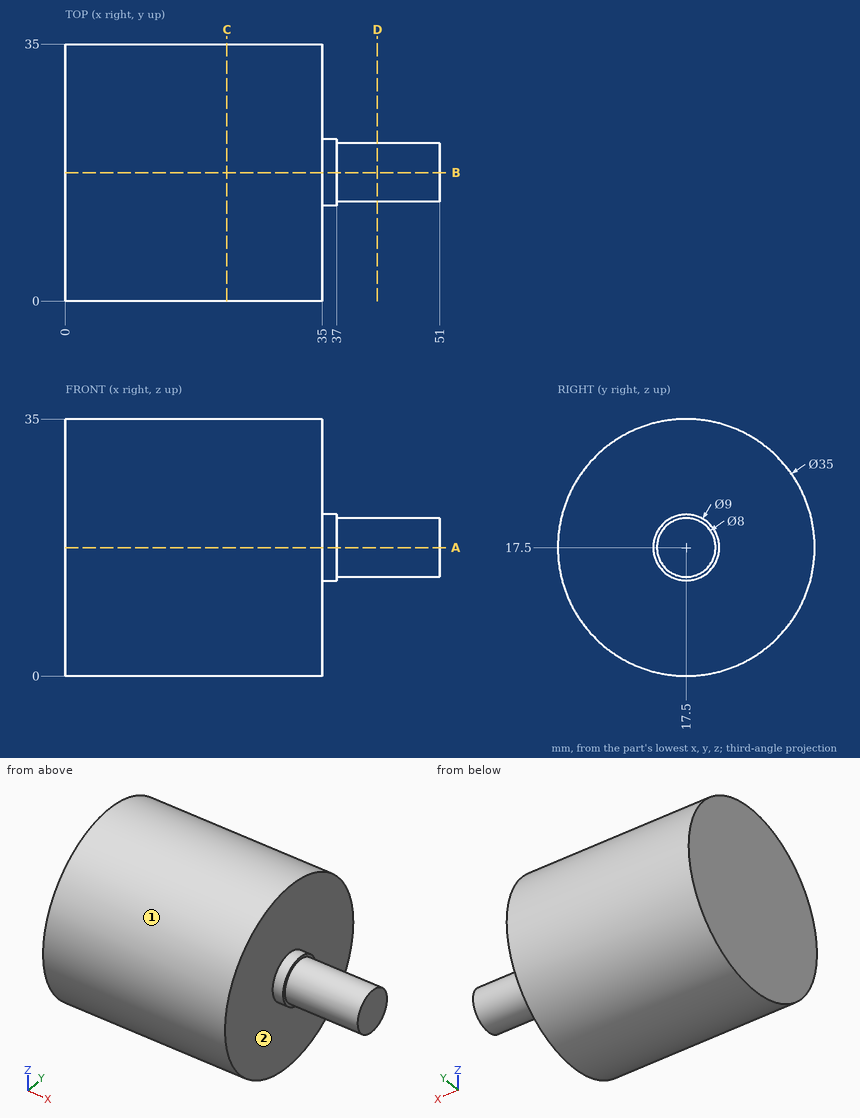
The drawing under review shows one solid part. Ordinate dimensions are in mm from its lowest x, y, z. A direction names the side the tool comes from. Give positions to 0.01 mm unless a question says otherwise; leave off trailing zeros. Loops run counter-clockwise (first coordinate to the right, second up) from the corner with the lowest first, then second, coordinate; pieces in that order, holes last. Notation, with made-up numbers: M -37,85 L -30,85 A11 ccw -30,98 Z; hole C 4,29.5 d10. An arc over 180 degrees is marked long. One line per item, written item: value. Start each with the question number.
Q1. Add section C-C (x = 22). Give the boundary of the cut face in (y, z), and give its area (3 significant figures).
Q2. Add section D-D (x = 42.5). Give the boundary of the cut face in (y, z).
Q3. Clearance check with flat-ended pins moving along their axes: pin 1 Ø10 at (x, z) = (32.5, 10.5) entering from -Y; pin 2 Ø2 at (x, z) = (9.5, 13) entering from +Y; pin 3 Ø1.5 at (x, z) = (29, 9.5) entering from +Y. State where each tip first meets the part, or that it passes through.
Q4. Machinability: for the marked faces 1 and 2, which of the approach directions +Z, -Z, +X, -X, +Y, -Y give a long, thin tool a straight path to every point of the face, cutting with its end or side? Answer none if there is none.
Q5. Add section A-A (z = 17.5). Give the boundary of the cut face in (x, y).
Q6. For L1, parallel to X at y = 9, z = 18.5; L2, parallel to Z at x = 28, y = 17; L3, parallel to Y at x = 5, z = 29.5, list the stretches that pass through material, from the lowest coordinate up.
Reply:
1. outline: C 17.5,17.5 d35
1. area: 962 mm²
2. outline: C 17.5,17.5 d8
3. pin 1: y = 0.11
3. pin 2: y = 34.65
3. pin 3: y = 33.43
4. face 1: +X, -X
4. face 2: +X
5. outline: M 0,0 L 35,0 L 35,13 L 37,13 L 37,13.5 L 51,13.5 L 51,21.5 L 37,21.5 L 37,22 L 35,22 L 35,35 L 0,35 Z
6. L1: 0 to 35
6. L2: 0.01 to 34.99
6. L3: 4.76 to 30.24
